Solid Edge part; units mm, degrees
sketch "Sketch1" plane through (0, 0, 0) normal (0, 0, 1) x (1, 0, 0)
  line L0 (-1.3856, 2.4) -> (1.3856, 2.4)
  line L1 (1.3856, 2.4) -> (2.7713, 0)
  line L2 (2.7713, 0) -> (1.3856, -2.4)
  line L3 (1.3856, -2.4) -> (-1.3856, -2.4)
  line L4 (-1.3856, -2.4) -> (-2.7713, 0)
  line L5 (-2.7713, 0) -> (-1.3856, 2.4)
extrude "Protrusion1" add sketch "Sketch1" along normal blind 0.5
sketch "Sketch2" plane through (0, 0, 0.5) normal (0, 0, 1) x (1, 0, 0)
  circle A0 centre (0, 0) radius 2.1
extrude "Ausprägung_2" add sketch "Sketch2" along normal blind 7.5
hole "Bohrung_1" at (0, 0, 8) direction (0, 0, -1) diameter 3 depth 5
chamfer "Fase_1" distance 0.2 angle 45 1 edges at (0, 1.5, 8)
Model file for the job. Use its own axes, mm. A direction names the side the tool comes from. Coordinates: 2 decimals unless noted, no trailing zeros. Write each loop counter-clockwise with the first axis right and the second up, starting at its lowest first coordinate (ties: lowest second). Pieces come first, ordered by that corner, then holes. Notation, with made-up numbers: (14.5, 41) - (47.5, 41) arc R27 ccw to (47.5, 69) - close; hole circle Ø9 at (33.25, -23). An arc over 180 degrees is marked (long way). Use a Markdown table: item, result. Add a question column.
Item 1: Band-saw the part on C-C, the plane z = 3.75. Write the cut outline in (x, y).
Item 2: Drill centre lines: line 1 along Y through (x, z) = (0, 6.05); line 2 along Z through (x, y) = (-0.85, 0.45); line 3 along X through (y, z) = (-0.4, 7). Where is each one in solid material? Low to high.
Item 3: Band-saw the part on A-A, the plane x = 0. Write the cut outline in (y, z).
Item 4: Band-saw the part on B-B, the plane z = 2. Write the cut outline in (x, y).
Item 5: Two-plate mould, pull along X, no slides. Class faces 3 (the face through (-2.09, 1.18, 0.25)), 4 (the face through (2.09, -1.18, 0.25)), 5 (the face through (-0.07, 1.5, 5.37)): pulls with the +X half, pulls with the -X half, needs draft (parallel to the pull), parting line crosses it, or undercut.
Item 6: 3-axis set-ups, long thin cutter, end or side, ignore diameter. For faces 1 (the face through (0, 0, 0)), 2 (the face through (0, 0, 3)): which of +Z, -Z, +X, -X, +Y, -Y reach the whole face in a straight line?
A:
| question | item | result |
|---|---|---|
| 1 | outline | circle Ø4.2 at (0, 0); hole circle Ø3 at (0, 0) |
| 2 | line 1 | y = -2.1 to -1.5, 1.5 to 2.1 |
| 2 | line 2 | z = 0 to 3 |
| 2 | line 3 | x = -2.06 to -1.45, 1.45 to 2.06 |
| 3 | outline | (-2.4, 0) - (2.4, 0) - (2.4, 0.5) - (2.1, 0.5) - (2.1, 8) - (1.7, 8) - (1.5, 7.8) - (1.5, 3) - (-1.5, 3) - (-1.5, 7.8) - (-1.7, 8) - (-2.1, 8) - (-2.1, 0.5) - (-2.4, 0.5) - close |
| 4 | outline | circle Ø4.2 at (0, 0) |
| 5 | face 3 | pulls with the -X half |
| 5 | face 4 | pulls with the +X half |
| 5 | face 5 | undercut |
| 6 | face 1 | -Z, +X, -X, +Y, -Y |
| 6 | face 2 | +Z |
